Input: part model. Units: mm. Frame: model coordinates. Face numbers are marked on the shaded views. A direction names the side the tool comes from. Coordinates: 2 decimals unless noted, no trailing zeros. Order: outer loops, then holes, each group sorted by start corner. A loop starts at its lowest first (then second) coordinate and runs counter-clockwise, first axis right, second up. Notation, with made-up numbers: (73, 8.5) -> (114, 8.5) arc R17 cw to (114, 18.5) -> close; hole circle Ø8 at (42, -6.75). An arc over 180 degrees is marked (long way). Answer as CSV lines item,"result".
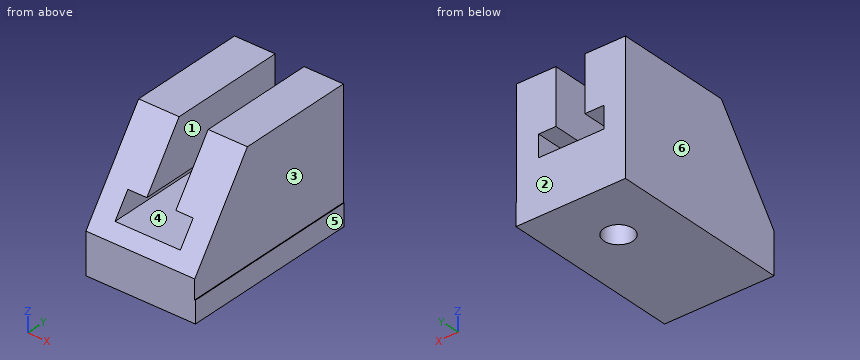
from build123d import *

# Parameters (mm, degrees)
F1_DEPTH = 25
F3_DEPTH = 18.7
F5_DEPTH = 3
F6_R     = 2
F7_DEPTH = 25


with BuildPart() as f1:
    # F0 (on Front) → F1 (new body)
    with BuildSketch(Plane.XZ):
        Polygon((-2.070283, 12.724239), (-7.654176, 12.724239), (-7.654176, -2.275761), (7.345824, -2.275761), (7.345824, 12.724239), (1.929717, 12.724239), (1.929717, 5.163504), (4.312236, 5.163504), (4.312236, 2.163504), (-4.687764, 2.163504), (-4.687764, 5.163504), (-2.070283, 5.163504), align=None)
        Polygon((7.345824, -2.275761), (-7.654176, -2.275761), (-7.654176, -5.275761), (7.44284, -5.275761), (7.44284, -2.275761), align=None)
    extrude(amount=F1_DEPTH)

    # F2 (on Right) → F3 (cut, symmetric)
    with BuildSketch(Plane.YZ):
        Polygon((-30.076236, 15.53787), (-27.17446, -2.654033), (-14.116468, 15.53787), align=None)
    extrude(amount=F3_DEPTH, both=True, mode=Mode.SUBTRACT)

    # F4 (on Top) → F5 (cut)
    with BuildSketch(Plane.XY):
        Polygon((3.278356, -9.464068), (2.653948, -6.020216), (-0.640718, -4.839043), (-3.310978, -7.101722), (-2.68657, -10.545573), (0.608097, -11.726746), align=None)
    extrude(amount=F5_DEPTH, mode=Mode.SUBTRACT)

    # F6 (on face) → F7 (cut)
    with BuildSketch(Plane.XY):
        with Locations((0, -8.177196)):
            Circle(F6_R)
    extrude(amount=-F7_DEPTH, mode=Mode.SUBTRACT)


solid = f1.part
1. Reachability of the marked faces 1, 2 and 3 from +Z, -Z, +X, -X, +Y, -Y: full face, straight path, thin tool, end or side. Return the list, or none.
Findings:
face 1,"+Z, +Y, -Y"
face 2,"+Z, -Z, +X, -X, +Y"
face 3,"+Z, +X, +Y, -Y"
2. Mould query, pull axis X, two halves, no side actions, for the marked faces 4, 5 and 6. Classes: released by +X, released by -X, zero draft, split by the parting line, or undercut.
Findings:
face 4,"undercut"
face 5,"released by +X"
face 6,"released by -X"
3. Cut plane A-A (x = 3.75). Return the cut outline in (y, z).
Findings:
outline,"(-25, -5.28) -> (0, -5.28) -> (0, 2.16) -> (-23.72, 2.16) -> (-25, 0.38) -> close; (-21.56, 5.16) -> (0, 5.16) -> (0, 12.72) -> (-16.14, 12.72) -> close"
4. Contact query for a flat-ended pin moving along its axis: pin 1 (4 mm diameter, centred on y = -6.5, z = 9, fed in from +X). Output: stop coordinate, or through.
Findings:
pin 1,"stops at x = 7.35"
5. Cut plane C-C (y = -2.25). Return the cut outline in (x, z), plus the area to 3 significant figures.
Findings:
outline,"(-7.65, -5.28) -> (7.44, -5.28) -> (7.44, -2.28) -> (7.35, -2.28) -> (7.35, 12.72) -> (1.93, 12.72) -> (1.93, 5.16) -> (4.31, 5.16) -> (4.31, 2.16) -> (-4.69, 2.16) -> (-4.69, 5.16) -> (-2.07, 5.16) -> (-2.07, 12.72) -> (-7.65, 12.72) -> close"
area,"213 mm2"
6. Ray query, line 1 along X through (y, z) = (-14.5, 6.25); line 2 along Y through (x, z) = (0, -3.95); line 3 along Z through (x, y) = (3.25, -5.25). Return the intervals inside material, ascending.
Findings:
line 1,"x = -7.65 to -2.07, 1.93 to 7.35"
line 2,"y = -25 to -10.18, -6.18 to 0"
line 3,"z = -5.28 to 2.16, 5.16 to 12.72"
7. Cut plane B-B (z = 7.75). Return the cut outline in (x, y).
Findings:
outline,"(-7.65, -19.71) -> (-2.07, -19.71) -> (-2.07, 0) -> (-7.65, 0) -> close; (1.93, -19.71) -> (7.35, -19.71) -> (7.35, 0) -> (1.93, 0) -> close"
8. Cut plane D-D (y = -9.75). Return the cut outline in (x, z).
Findings:
outline,"(-7.65, -5.28) -> (-1.24, -5.28) -> (-1.24, 0) -> (-2.83, 0) -> (-2.83, 2.16) -> (-4.69, 2.16) -> (-4.69, 5.16) -> (-2.07, 5.16) -> (-2.07, 12.72) -> (-7.65, 12.72) -> close; (1.24, -5.28) -> (7.44, -5.28) -> (7.44, -2.28) -> (7.35, -2.28) -> (7.35, 12.72) -> (1.93, 12.72) -> (1.93, 5.16) -> (4.31, 5.16) -> (4.31, 2.16) -> (2.94, 2.16) -> (2.94, 0) -> (1.24, 0) -> close"
